Here's the drawing with two shaded views (mm, measured from the low corner). I have some questions. Give positions to 0.01 mm unless a question says otherwise; leave off trailing zeros. Order: outer loops, then holes, each group sorted by start corner. A loop starts at its lowest first (then second) coordinate and runs counter-clockwise, first axis right, second up. Notation, with made-up numbers: M 21,80.5 L 63,80.5 A10 cw 63,99.5 Z; hole C 3,-13 d2. An arc over 180 degrees is marked long. One line per question, with ' | ' between items. Start each with the question number.
1) If we section it at A-A, the plane z = 61: Please give me the cut outline in (x, y).
2) If we section it at D-D, the plane x = 178.5: Please give me the cut outline in (y, z).
3) Please list where these lines run through material, in increasing order: line 1 along X through (y, z) = (2.85, 61); line 2 along Z through (x, y) = (199, 1.7); line 3 along Z through (x, y) = (32, 3.2). Write a range as [from, to].
4) If we section it at B-B, the plane x = 21: Please give me the cut outline in (y, z).
5) I'm going to push flat-ended pins straight in: pin 1 Ø3 at (y, z) = (3, 79) entering from +X; pin 2 Ø1 at (y, z) = (1.5, 49.5) entering from +X; pin 3 Ø1 at (y, z) = (5.5, 41) entering from -X. Where does each tip first touch, or does it pass through?
6) If we section it at C-C, the plane y = 3.35: State how many separate pieces and enclosed holes the cut face has, plus the area to 3 significant figures.
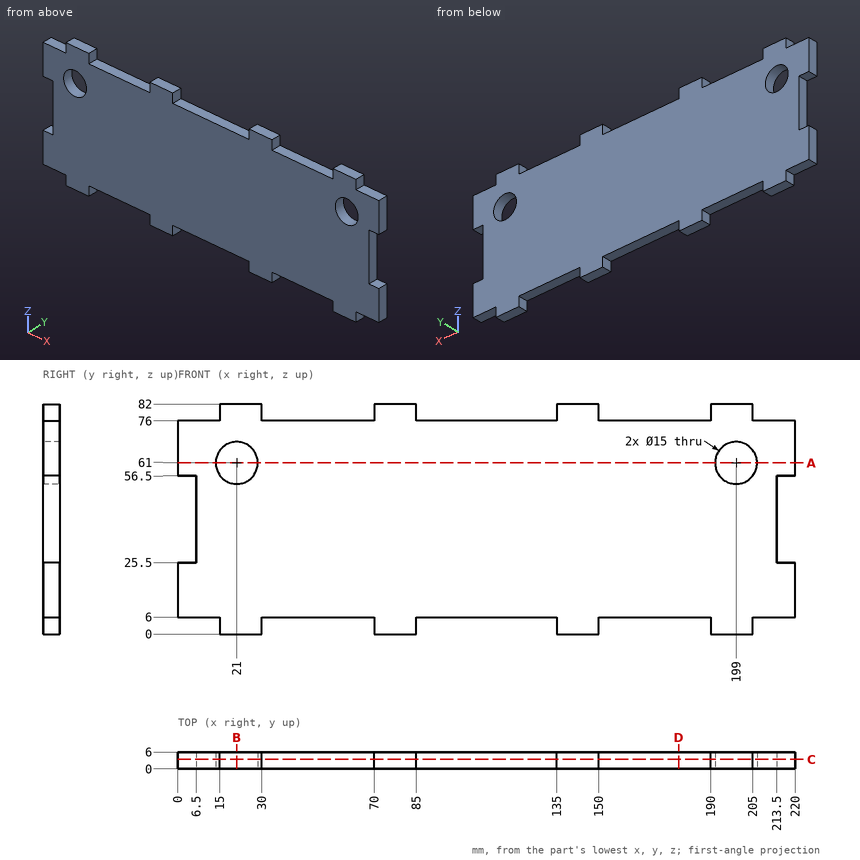
Results found:
1) outline: M 0,0 L 13.5,0 L 13.5,6 L 0,6 Z; M 28.5,0 L 191.5,0 L 191.5,6 L 28.5,6 Z; M 206.5,0 L 220,0 L 220,6 L 206.5,6 Z
2) outline: M 0,6 L 6,6 L 6,76 L 0,76 Z
3) line 1: x = [0, 13.5], [28.5, 191.5], [206.5, 220] | line 2: z = [0, 53.5], [68.5, 82] | line 3: z = [6, 76]
4) outline: M 0,0 L 6,0 L 6,53.5 L 0,53.5 Z; M 0,68.5 L 6,68.5 L 6,82 L 0,82 Z
5) pin 1: stops at x = 205 | pin 2: stops at x = 213.5 | pin 3: stops at x = 6.5
6) separate pieces: 1 | enclosed holes: 2 | area: 15,400 mm²
